```python
from build123d import *

# Parameters (mm, degrees)
SKETCH1_R           = 6.901519969
SKETCH1_R_2         = 6.9
SKETCH1_R_3         = 2.6
BOSS_EXTRUDE1_DEPTH = 5
SKETCH2_R           = 4
SKETCH2_R_2         = 2.6
BOSS_EXTRUDE2_DEPTH = 2
SCALE1_SCALE        = 1.5


with BuildPart() as part:
    # Sketch1 → Boss-Extrude1 (new body)
    with BuildSketch(Plane.XY):
        with BuildLine():
            Line((-119.047770685, -14.21840763), (-158.491736924, 19.646141241))
            add(Edge.make_bspline(
                [(-158.491736924, 19.646141241), (-160.313597407, 21.050397122), (-161.909962094, 22.656519407)],
                knots=[0, 0, 0, 1, 1, 1], degree=2))
            ThreePointArc((-161.909962094, 22.656519407), (-163.491640093, 26.517106064), (-166.64545249, 29.248278339))
            Line((-166.64545249, 29.248278339), (-169.551288031, 37.112526103))
            ThreePointArc((-169.551288031, 37.112526103), (-180.421756419, 49.833075564), (-181.222431589, 33.119656379))
            Line((-181.222431589, 33.119656379), (-178.794316039, 25.37582765))
            ThreePointArc((-178.794316039, 25.37582765), (-178.212831269, 16.189990788), (-169.857983808, 12.328093938))
            Line((-169.857983808, 12.328093938), (-127.253789064, -21.937441374))
            ThreePointArc((-127.253789064, -21.937441374), (-117.207191003, -24.396487309), (-119.047770685, -14.21840763))
        make_face()
        with Locations((-170.794274728, 21.270925714)):
            Circle(SKETCH1_R, mode=Mode.SUBTRACT)
        with Locations((-177.508495403, 41.317624299)):
            Circle(SKETCH1_R_2, mode=Mode.SUBTRACT)
        with Locations((-121.432089481, -19.905045023)):
            Circle(SKETCH1_R_3, mode=Mode.SUBTRACT)
    extrude(amount=BOSS_EXTRUDE1_DEPTH)

    # Sketch2 → Boss-Extrude2 (add)
    with BuildSketch(Plane.XY.offset(5)):
        with BuildLine():
            Line((-119.047770685, -14.21840763), (-158.491736924, 19.646141241))
            add(Edge.make_bspline(
                [(-158.491736924, 19.646141241), (-160.313597387, 21.050397106), (-161.909962058, 22.656519371)],
                knots=[0, 0, 0, 1, 1, 1], degree=2))
            ThreePointArc((-161.909962058, 22.656519371), (-163.491640057, 26.517106064), (-166.64545249, 29.248278339))
            Line((-166.64545249, 29.248278339), (-169.551288031, 37.112526103))
            ThreePointArc((-169.551288031, 37.112526103), (-180.421756419, 49.833075564), (-181.222431589, 33.119656379))
            Line((-181.222431589, 33.119656379), (-178.794316039, 25.37582765))
            ThreePointArc((-178.794316039, 25.37582765), (-178.212831269, 16.189990788), (-169.857983808, 12.328093938))
            Line((-169.857983808, 12.328093938), (-127.253789064, -21.937441374))
            ThreePointArc((-127.253789064, -21.937441374), (-117.207191003, -24.396487309), (-119.047770685, -14.21840763))
        make_face()
        with Locations((-177.508495403, 41.317624299)):
            Circle(SKETCH2_R, mode=Mode.SUBTRACT)
        with Locations((-170.794274728, 21.270925714)):
            Circle(SKETCH2_R, mode=Mode.SUBTRACT)
        with Locations((-121.432089481, -19.905045023)):
            Circle(SKETCH2_R_2, mode=Mode.SUBTRACT)
    extrude(amount=BOSS_EXTRUDE2_DEPTH)


with BuildPart() as part_1:
    # Scale1: scaled about (-152.018458466, 8.096190601, 3.636452689)
    add(part.part.scale(SCALE1_SCALE).moved(Location((76.009229233, -4.0480953, -1.818226344))))


solid = part_1.part
```
Input: part model. Units: mm. Frame: model coordinates. A direction names the side the tool comes from. Coordinates: 2 decimals unless noted, no trailing zeros. Loops run counter-clockwise (first coordinate to the right, second up) from the corner with the lowest first, then second, coordinate; pieces in that order, holes last. Notation, with made-up numbers: M -19,-15.5 L 0,-15.5 A5 ccw 0,-9.5 Z; hole C -16,-34.75 d10. An arc over 180 degrees is marked long. One line per item, written item: value.
(1) Section A-A (y = 32). Output: boundary loops of the cut face in (x, z), and give its area (3 significant figures).
Filled in:
outline: M -193.02,-1.82 L -189.67,-1.82 L -189.67,5.68 L -184.52,5.68 L -184.52,8.68 L -193.02,8.68 Z; M -175.84,5.68 L -170.69,5.68 L -170.69,-1.82 L -167.35,-1.82 L -167.35,8.68 L -175.84,8.68 Z
area: 101 mm^2
(2) Reachability of faces 5 (the flat face through (-186, 53, 5.682)), 6 (the flat face through (-151, 6, -1.818)), 7 (the cylindrical face through (-194.19, 70.84, 3.36)), 8 (the flat face through (-194.029, 39.905, 3.358)), 9 (the flat face through (-176.108, 45.64, 3.358)) from +Z, -Z, +X, -X, +Y, -Y: full face, straight path, thin tool, end or side. Return the list, or none.
Filled in:
face 5: -Z
face 6: -Z, +X, -X, +Y, -Y
face 7: +Z, -Z
face 8: +Z, -Z, -X
face 9: +Z, -Z, +X
(3) Section D-D (z = 0.5). Give the number of separate pieces and of enclosed holes in the cut face, and give its area (3 significant figures).
Filled in:
separate pieces: 1
enclosed holes: 3
area: 2,210 mm^2
(4) Line query: line 1 along Y through (x, z) = (-187.5, 7.25); line 2 along X through (y, z) = (23.5, 2.75); line 3 along Y through (x, z) = (-191.5, 4.5). Output: solid intervals per line, ascending. Write a range as from..to.
Filled in:
line 1: 16.53..52.6, 63.26..71.14
line 2: -192.95..-189.57, -170.79..-159.49
line 3: 20.52..47.65, 68.2..71.37
(5) Section C-C (x = -128.5). Output: boundary loops of the cut face in (y, z).
Filled in:
outline: M -25.99,-1.82 L -3.11,-1.82 L -3.11,8.68 L -25.99,8.68 Z
(6) Section B-B (y = 54.5). Output: boundary loops of the cut face in (x, z), and give its area (3 significant figures).
Filled in:
outline: M -203.31,-1.82 L -200.02,-1.82 L -200.02,5.68 L -195.18,5.68 L -195.18,8.68 L -203.31,8.68 Z; M -185.33,5.68 L -180.49,5.68 L -180.49,-1.82 L -177.2,-1.82 L -177.2,8.68 L -185.33,8.68 Z
area: 98.2 mm^2
(7) Pull-direction query (Y, two-part tool) for faces 1 (the cylindrical face through (-99.992, -40.817, 3.358)), 2 (the cylindrical face through (-191.423, 20.405, 3.358)), 3 (the flat face through (-131.731, -0.333, 3.358)), 4 (the flat face through (-155, 10, 8.682)); classes: +Y half, -Y half, draft (parallel to the pull), parting line (faces both ways), or undercut.
Filled in:
face 1: parting line
face 2: undercut
face 3: +Y half
face 4: draft
(8) Pin query (flat end, axial travel): pin 1 (4 mm diameter, centred on y = 42, z = -0.5, fed in from -X); pin 2 (6 mm diameter, centred on x = -106.14, y = -33.91, fed in from -Z); pin 3 (5 mm diameter, centred on x = -168, z = 7, fed in from +Y); pin 4 (1.5 mm diameter, centred on x = -119.5, z = 2.5, fed in from +Y). Return the tip coordinate at first contact, or that it passes through.
Filled in:
pin 1: x = -195.31
pin 2: through
pin 3: y = 37.25
pin 4: y = -10.19
